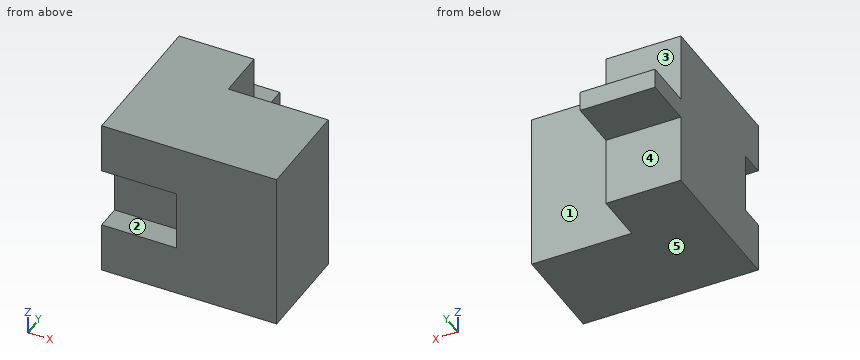
from build123d import *

# Parameters (mm, degrees)
BOSS_EXTRUDE1_DEPTH = 32
SKETCH2_W           = 14
SKETCH2_H           = 10
SKETCH2_W_2         = 12
CUT_EXTRUDE1_DEPTH  = 51.049529889


with BuildPart() as part:
    # Sketch1 → Boss-Extrude1 (new body)
    with BuildSketch(Plane.XY):
        Polygon((-36.032249566, 32.877886825), (-51.032249566, 32.877886825), (-51.032249566, -7.122113175), (-16.032249566, -7.122113175), (-16.032249566, 12.877886825), (-36.032249566, 12.877886825), align=None)
    extrude(amount=BOSS_EXTRUDE1_DEPTH)

    # Sketch2 → Cut-Extrude1 (cut, through all)
    with BuildSketch(Plane(origin=(-36.032249566, 0, 0), x_dir=(0, 0, -1), z_dir=(1, 0, 0))):
        with Locations((-7, 27.877886825)):
            Rectangle(SKETCH2_W, SKETCH2_H)
        with Locations((-25, 27.877886825)):
            Rectangle(SKETCH2_W, SKETCH2_H)
        with Locations((-16, -7.122113175)):
            Rectangle(SKETCH2_W_2, SKETCH2_H)
    extrude(amount=-CUT_EXTRUDE1_DEPTH, mode=Mode.SUBTRACT)


solid = part.part
Work out the finished part from the listing and answer in its coordinate system (mm). Face numbers are marked on the shaded views. A direction names the side the tool comes from. Round coordinates to 2 decimals unless told otherwise and drop trailing zeros. Write each loop counter-clockwise with the first axis right and the second up, starting at its lowest first coordinate (ties: lowest second). Pieces come first, ordered by that corner, then holes.
1) Given pin 1 Ø3 at (x, y) = (-41.5, 28.5) entering from -Z; pin 2 Ø7 at (x, z) = (-42, 26) entering from +Y; pin 3 Ø16 at (x, z) = (-27, 9) entering from +Y; pin 4 Ø1.5 at (x, y) = (-21, 14.5) entering from +Z, each flat-ended and moving along its own axis, determine where each tip first touches the part or whether it passes through.
2) A cutting plane is placed at A-A (z = 19.5). Give the vertices of the cut face in (x, y), plus the area to 3 significant figures.
3) A cutting plane is placed at C-C (y = -5). Give the vertices of the cut face in (x, z), plus the area to 3 significant figures.
4) Straight lines are drawn through the part: line 1 (Z direction, x = -38.5, y = -4); line 2 (Y direction, x = -27, z = 4); line 3 (Z direction, x = -46.5, y = 23.5). For each, find the intervals that lie inside material, in ascending order.
5) A cutting plane is placed at B-B (x = -37.5). Give the vertices of the cut face in (y, z), plus the area to 3 significant figures.
6) A tool of negligible diameter and unlimited length cuts with its end or side. For the marked faces 1, 2, 3, 4 and 5, from which of +Z, -Z, +X, -X, +Y, -Y can it reach the whole face along a straight path? Write none if from no direction.
7) A cutting plane is placed at D-D (z = 3.5). Give the vertices of the cut face in (x, y), plus the area to 3 significant figures.
Completed:
1. pin 1: stops at z = 14
1. pin 2: stops at y = 22.88
1. pin 3: stops at y = 12.88
1. pin 4: passes through
2. outline: (-51.03, -2.12) - (-36.03, -2.12) - (-36.03, -7.12) - (-16.03, -7.12) - (-16.03, 12.88) - (-36.03, 12.88) - (-36.03, 22.88) - (-51.03, 22.88) - close
2. area: 775 mm2
3. outline: (-51.03, 0) - (-16.03, 0) - (-16.03, 32) - (-51.03, 32) - (-51.03, 22) - (-36.03, 22) - (-36.03, 10) - (-51.03, 10) - close
3. area: 940 mm2
4. line 1: z = 0 to 10, 22 to 32
4. line 2: y = -7.12 to 12.88
4. line 3: z = 14 to 18
5. outline: (-7.12, 0) - (22.88, 0) - (22.88, 14) - (32.88, 14) - (32.88, 18) - (22.88, 18) - (22.88, 32) - (-7.12, 32) - (-7.12, 22) - (-2.12, 22) - (-2.12, 10) - (-7.12, 10) - close
5. area: 940 mm2
6. face 1: +Z, -Z, +X, +Y
6. face 2: -X, -Y
6. face 3: +Z, +X, -X, +Y
6. face 4: -Z, +X, -X, +Y
6. face 5: -Z, +X, -X, +Y, -Y
7. outline: (-51.03, -7.12) - (-16.03, -7.12) - (-16.03, 12.88) - (-36.03, 12.88) - (-36.03, 22.88) - (-51.03, 22.88) - close
7. area: 850 mm2
